```python
from build123d import *

# Parameters (mm, degrees)
SKETCH2_W           = 22.225
SKETCH2_H           = 1066.8
BOSS_EXTRUDE1_DEPTH = 12.7
SKETCH3_W           = 9.525
SKETCH3_H           = 12.7
CUT_EXTRUDE1_DEPTH  = 1067.933464494
CUT_EXTRUDE2_DEPTH  = 535.120031132


with BuildPart() as part:
    # Sketch2 → Boss-Extrude1 (new, symmetric)
    with BuildSketch(Plane.XY):
        Rectangle(SKETCH2_W, SKETCH2_H)
    extrude(amount=BOSS_EXTRUDE1_DEPTH, both=True)

    # Sketch3 → Cut-Extrude1 (cut, through all)
    with BuildSketch(Plane(origin=(0, 533.4, 0), x_dir=(1, 0, 0), z_dir=(0, 1, 0))):
        Rectangle(SKETCH3_W, SKETCH3_H)
    extrude(amount=-CUT_EXTRUDE1_DEPTH, mode=Mode.SUBTRACT)

    # Sketch4 → Cut-Extrude2 (cut, through all)
    with BuildSketch(Plane.XY.offset(12.7)):
        Polygon((11.1125, 533.4), (-11.1125, 514.751010697), (-11.1125, 533.4), align=None)
    extrude(amount=-CUT_EXTRUDE2_DEPTH, mode=Mode.SUBTRACT)


solid = part.part
```
Geometry: final body of the model. Coordinates: model frame, mm. Coordinates: 2 decimals unless noted, no trailing zeros. Order: outer loops, then holes, each group sorted by start corner. A loop starts at its lowest first (then second) coordinate and runs counter-clockwise, first axis right, second up. Notation, with made-up numbers: M 65,18.5 L 100,18.5 A21 cw 100,56.5 Z; hole C -37,21 d11. An arc over 180 degrees is marked long. Answer in a Markdown table with one row per item. Add a question column.
Q1. Section query B-B on y = -32. Return the cut outline in (x, z).
Q2. Mould query, pull axis X, two halves, no side actions, for faces 1 (the flat face through (11.112, -7, 0)), 2 (the flat face through (-11.112, -17, 0)), 3 (the flat face through (0, 7, -12.7)). Classes: released by +X, released by -X, zero draft, split by the parting line, or undercut.
Q3. Section query A-A on z = -0.75. Return the cut outline in (x, y).
Q4. Contact query for a flat-ended pin moving along its axis: P1, Ø10, axis at x = -2.5, z = 4, coming from the +Y side. Output: stop coordinate, or through.
Q5. Line query: L1, parallel to Z at x = 2.5, y = 54; L2, parallel to X at y = -441, z = 5.5; L3, parallel to Y at x = -5, z = 5.5. Output: solid intervals per line, ascending.
Completed:
| question | item | result |
|---|---|---|
| 1 | outline | M -11.11,-12.7 L 11.11,-12.7 L 11.11,12.7 L -11.11,12.7 Z; hole M -4.76,-6.35 L 4.76,-6.35 L 4.76,6.35 L -4.76,6.35 Z |
| 2 | face 1 | released by +X |
| 2 | face 2 | released by -X |
| 2 | face 3 | zero draft |
| 3 | outline | M -11.11,-533.4 L -4.76,-533.4 L -4.76,520.08 L -11.11,514.75 Z; M 4.76,-533.4 L 11.11,-533.4 L 11.11,533.4 L 4.76,528.07 Z |
| 4 | P1 | stops at y = 525.68 |
| 5 | L1 | z = -12.7 to -6.35, 6.35 to 12.7 |
| 5 | L2 | x = -11.11 to -4.76, 4.76 to 11.11 |
| 5 | L3 | y = -533.4 to 519.88 |
